Autodesk Inventor part; units mm, degrees
ref_plane "YZ Plane" through (0, 0, 0) normal (1, 0, 0) x (0, 1, 0)
ref_plane "XZ Plane" through (0, 0, 0) normal (0, 1, 0) x (-1, 0, 0)
ref_plane "XY Plane" through (0, 0, 0) normal (0, 0, 1) x (1, 0, 0)
sketch "Sketch1" plane through (0, 0, 0) normal (0, 1, 0) x (-1, 0, 0)
  line L0 (69.75, 45) -> (-69.75, 45)
  line L1 (-69.75, 45) -> (-69.75, -45)
  line L2 (-69.75, -45) -> (69.75, -45)
  line L3 (69.75, -45) -> (69.75, 45)
  line L4 (69.75, 45) -> (-69.75, -45) construction
  line L5 (-69.75, 45) -> (69.75, -45) construction
  circle A0 centre (-15.25, 0) radius 14.5
  line L6 (152.1746, 0) -> (-152.1746, 0) construction
  line L7 (0, 58.0523) -> (0, -58.0523) construction
  point P0 (0, 0)
  dimension "d0" = 139.5
  dimension "d2" = 29
  dimension "d4" = 90
  dimension "d5" = 54.5
extrude "Extrusion1" add sketch "Sketch1" along normal blind 10
sketch "Sketch2" plane through (0, 10, 0) normal (0, 1, 0) x (1, 0, 0)
  line L0 (-64.75, -40) -> (64.75, -40) construction
  line L1 (64.75, -40) -> (64.75, 40) construction
  line L2 (64.75, 40) -> (-64.75, 40) construction
  line L3 (-64.75, 40) -> (-64.75, -40) construction
  line L4 (-64.75, -40) -> (64.75, 40) construction
  line L5 (64.75, -40) -> (-64.75, 40) construction
  line L6 (69.75, 45) -> (-69.75, 45)
  line L7 (69.75, -45) -> (69.75, 45)
  point P0 (0, 0)
  dimension "d11" = 5
  dimension "d12" = 5
hole "Hole1" at (-64.75, 10, -40) at (64.75, 10, -40) at (64.75, 10, 40) at (-64.75, 10, 40) direction (0, -1, 0) diameter 3.4 end through all counterbore diameter 6.5 counterbore depth 3.4
sketch "Sketch3" plane through (0, 0, 0) normal (0, -1, 0) x (1, 0, 0)
  circle A0 centre (-64.75, 40) radius 3.25
  circle A1 centre (-64.75, 40) radius 4
  circle A2 centre (-64.75, 40) radius 1.7
  circle A3 centre (64.75, 40) radius 1.7
  circle A4 centre (64.75, -40) radius 1.7
  circle A5 centre (-64.75, -40) radius 1.7
  line L0 (69.75, 45) -> (69.75, -45)
  line L1 (-69.75, 45) -> (69.75, 45)
  line L2 (-69.75, -45) -> (-69.75, 45)
  line L3 (69.75, -45) -> (-69.75, -45)
  circle A6 centre (64.75, 40) radius 4
  circle A7 centre (-64.75, -40) radius 4
  circle A8 centre (64.75, -40) radius 4
  point P0 (0, 0)
  dimension "d22" = 129.5
  dimension "d25" = 80
  dimension "d28" = 8
  dimension "d63" = 90
  dimension "d64" = 139.5
extrude "Extrusion2" cut sketch "Sketch3" against normal blind 1 contours A0 | A1 | A2 | A3 | A4 | A5 | A6 | A7 | A8
sketch "Sketch4" plane through (0, 0, 0) normal (0, -1, 0) x (1, 0, 0)
  circle A0 centre (64.75, -40) radius 4
  circle A1 centre (-64.75, -40) radius 4
  circle A2 centre (64.75, 40) radius 4
  circle A3 centre (-64.75, 40) radius 4
  line L0 (69.75, 45) -> (69.75, -45)
  line L1 (-69.75, 45) -> (69.75, 45)
  line L2 (-69.75, -45) -> (-69.75, 45)
  line L3 (69.75, -45) -> (-69.75, -45)
  circle A4 centre (15.25, 0) radius 14.5
  circle A5 centre (15.25, 0) radius 17.5
  point P0 (0, 0)
  dimension "d31" = 35
extrude "Extrusion3" cut sketch "Sketch4" against normal blind 5 contours A5
sketch "Sketch5" plane through (0, 0, 0) normal (0, -1, 0) x (1, 0, 0)
  line L0 (-59.75, 45) -> (-29.75, 45) construction
  line L1 (-29.75, 45) -> (-29.75, -45) construction
  line L2 (-29.75, -45) -> (-59.75, -45) construction
  line L3 (-59.75, -45) -> (-59.75, 45) construction
  line L4 (-97.65, 0) -> (97.65, 0)
  circle A0 centre (-54.75, 40) radius 4
  circle A1 centre (-34.75, 40) radius 4
  circle A2 centre (-54.75, -40) radius 4
  circle A3 centre (-34.75, -40) radius 4
  line L5 (-59.75, 45) -> (-29.75, -45) construction
  line L6 (-69.75, -45) -> (-69.75, 45)
  point P0 (0, 0)
  point P1 (-59.75, 0)
  point P2 (-44.75, 0)
  dimension "d34" = 90
  dimension "d35" = 30
  dimension "d36" = 8
  dimension "d37" = 5
  dimension "d38" = 5
  dimension "d41" = 20
  dimension "d44" = 80
  dimension "d47" = 25
  dimension "d65" = 90
extrude "Extrusion4" cut sketch "Sketch5" against normal blind 1
sketch "Sketch7" plane through (0, 10, 0) normal (0, 1, 0) x (1, 0, 0)
  circle A0 centre (-54.75, -40) radius 4 construction
  point P0 (0, 0)
hole "Hole2" at (-54.75, 10, 40) direction (0, -1, 0) diameter 3.4 end through all counterbore diameter 6.5 counterbore depth 3.4
pattern_linear "Rectangular Pattern1" count 2 spacing 80 along (0, 0, -1) count 2 spacing 20 along (1, 0, 0) of "Hole2"
sketch "Sketch8" plane through (0, 10, 0) normal (0, 1, 0) x (1, 0, 0)
  circle A0 centre (-34.75, 40) radius 3.25
  circle A1 centre (-34.75, -40) radius 3.25
  circle A2 centre (-54.75, 40) radius 3.25
  circle A3 centre (-54.75, -40) radius 3.25
  circle A4 centre (-64.75, -40) radius 3.25
  circle A5 centre (64.75, -40) radius 3.25
  circle A6 centre (64.75, 40) radius 3.25
  circle A7 centre (-64.75, 40) radius 3.25
  line L0 (69.75, -45) -> (69.75, 45)
  line L1 (69.75, 45) -> (-69.75, 45)
  line L2 (-69.75, 45) -> (-69.75, -45)
  line L3 (-69.75, -45) -> (69.75, -45)
  circle A8 centre (15.25, 0) radius 14.5
  circle A9 centre (15.25, 0) radius 9
  point P0 (0, 0)
  dimension "d66" = 18
extrude "Extrusion5" add sketch "Sketch8" against normal blind 4 contours A8
sketch "Sketch9" plane through (0, 10, 0) normal (0, 1, 0) x (1, 0, 0)
  circle A0 centre (15.25, 0) radius 9
  circle A1 centre (-34.75, 40) radius 3.25
  circle A2 centre (-34.75, -40) radius 3.25
  circle A3 centre (-54.75, 40) radius 3.25
  circle A4 centre (-54.75, -40) radius 3.25
  circle A5 centre (-64.75, -40) radius 3.25
  circle A6 centre (64.75, -40) radius 3.25
  circle A7 centre (64.75, 40) radius 3.25
  circle A8 centre (-64.75, 40) radius 3.25
  line L0 (69.75, -45) -> (69.75, 45)
  line L1 (69.75, 45) -> (-69.75, 45)
  line L2 (-69.75, 45) -> (-69.75, -45)
  line L3 (-69.75, -45) -> (69.75, -45)
  line L4 (-79.75, 55) -> (79.75, 55)
  line L5 (79.75, 55) -> (79.75, -55)
  line L6 (79.75, -55) -> (-79.75, -55)
  line L7 (-79.75, -55) -> (-79.75, 55)
  point P0 (0, 0)
  dimension "d69" = 10
  dimension "d70" = 10
  dimension "d71" = 10
  dimension "d72" = 10
extrude "Extrusion6" add sketch "Sketch9" against normal blind 4 contours L4 L5 L6 L7
fillet "Fillet1" radius 2 8 edges at (-79.75, 8, 55) (-69.75, 3, 45) (69.75, 3, 45) (79.75, 8, 55) (79.75, 8, -55) (69.75, 3, -45) (-69.75, 3, -45) (-79.75, 8, -55)
sketch "Sketch11" plane through (0, 10, 0) normal (0, 1, 0) x (1, 0, 0)
  line L0 (74.75, -50) -> (-74.75, -50) construction
  line L1 (-74.75, -50) -> (-74.75, 50) construction
  line L2 (-74.75, 50) -> (74.75, 50) construction
  line L3 (74.75, 50) -> (74.75, -50) construction
  line L4 (-79.75, 53) -> (-79.75, -53) construction
  line L5 (77.75, 55) -> (-77.75, 55) construction
  line L6 (-77.75, -55) -> (77.75, -55) construction
  line L7 (79.75, -53) -> (79.75, 53) construction
  point P0 (0, 0)
  dimension "d87" = 5
  dimension "d88" = 5
  dimension "d89" = 5
  dimension "d90" = 5
hole "Hole4" at (-74.75, 10, 50) at (-74.75, 10, -50) at (74.75, 10, -50) at (74.75, 10, 50) direction (0, -1, 0) diameter 3.4 end through all
equation "\"d34\" = d65"
properties part number "plate 2 for print"
Could you check a few things on this model? Use its own coordinates, in mm. A direction names the side the tool comes from. Give positions to 0.01 mm unless a question says otherwise; leave off trailing zeros. Order: outer loops, then holes, each group sorted by start corner. A loop starts at its lowest first (then second) coordinate and runs counter-clockwise, first axis right, second up.
Item 1: For faces 1 (the face through (63.6, 3.76, 38.75)), 2 (the face through (-33, 6.6, 41)), 3 (the face through (-60.935, 0.493, 41.201)), which set-ups out of +Z, -Z, +X, -X, +Y, -Y let a thin tool reach every point of the face, with its end or its side?
Item 2: If we section it at B-B, the plane z = -50: Write out the boundary of the cut face in (x, y).
Item 3: I'm going to push flat-ended pins straight in: pin 1 (4.5 mm diameter, centred on x = -64.75, z = 40, fed in from -Y); pin 2 (1.5 mm diameter, centred on y = 1.5, z = 9.5, fed in from -X); pin 3 (2 mm diameter, centred on x = -34, z = 41.5, fed in from +Y). Where does each tip first touch, or does it pass through?
Item 4: I need wall thicknesses on line 1 (X direction, y = 8.7, z = 40); line 2 (X direction, y = 4.5, z = 40); line 3 (Z direction, x = -64.75, y = 0.35). Which ranges of each line are inside material? Lowest first, please.
Item 5: If we mould it in two halves opening along X, with no side actions, what happens to faces 4 (the face through (-1, 10, -1)), 5 (the face through (-55, 1, -42)), 6 (the face through (-69.75, 3, -1))? For each: pulls with the +X half, pulls with the -X half, needs draft (parallel to the pull), parting line crosses it, or undercut.
Item 6: If we section it at C-C, the plane z = 0: Write out the boundary of the cut face in (x, y).
Item 7: If we section it at D-D, the plane x = 15.25: Write out the boundary of the cut face in (y, z), plus the area to 3 significant figures.
Item 8: If we section it at A-A, the plane x = 64.75: Count the separate pieces of the cut face and the enclosed holes in it, plus the area to 3 significant figures.
Values:
1. face 1: +Y, -Y
1. face 2: +Y
1. face 3: -Y
2. outline: (-79.75, 6) - (-76.45, 6) - (-76.45, 10) - (-79.75, 10) - close; (-73.05, 6) - (73.05, 6) - (73.05, 10) - (-73.05, 10) - close; (76.45, 6) - (79.75, 6) - (79.75, 10) - (76.45, 10) - close
3. pin 1: stops at y = 1
3. pin 2: stops at x = -69.75
3. pin 3: stops at y = 6.6
4. line 1: x = -79.75 to -68, -61.5 to -58, -51.5 to -38, -31.5 to 61.5, 68 to 79.75
4. line 2: x = -69.75 to -66.45, -63.05 to -56.45, -53.05 to -36.45, -33.05 to 63.05, 66.45 to 69.75
4. line 3: z = -45 to -44, -36 to 36, 44 to 45
5. face 4: needs draft
5. face 5: undercut
5. face 6: pulls with the -X half
6. outline: (-79.75, 6) - (-69.75, 6) - (-69.75, 0) - (-2.25, 0) - (-2.25, 5) - (0.75, 5) - (0.75, 6) - (6.25, 6) - (6.25, 10) - (-79.75, 10) - close; (24.25, 6) - (29.75, 6) - (29.75, 5) - (32.75, 5) - (32.75, 0) - (69.75, 0) - (69.75, 6) - (79.75, 6) - (79.75, 10) - (24.25, 10) - close
7. outline: (0, -45) - (6, -45) - (6, -55) - (10, -55) - (10, -9) - (6, -9) - (6, -14.5) - (5, -14.5) - (5, -17.5) - (0, -17.5) - close; (0, 17.5) - (5, 17.5) - (5, 14.5) - (6, 14.5) - (6, 9) - (10, 9) - (10, 55) - (6, 55) - (6, 45) - (0, 45) - close
7. area: 704 mm2
8. separate pieces: 3
8. enclosed holes: 0
8. area: 882 mm2
